For this review, take the finished solid that the model builds, in its own axes (mm). A direction names the side the tool comes from. Round coordinates to 2 decimals unless told otherwise and drop trailing zeros. Order: outer loops, then holes, each group sorted by start corner. A loop starts at its lowest first (then second) coordinate and runs counter-clockwise, first axis right, second up.
from build123d import *

# Parameters (mm, degrees)
SKETCH1_R                   = 5
SKETCH1_R_2                 = 1.15
BOSS_EXTRUDE1_DEPTH         = 1.5
FILLET1_R                   = 3
TAP_DRILL_FOR_M2_TAP1_D     = 1.6
TAP_DRILL_FOR_M2_TAP1_DEPTH = 6
TAP_DRILL_FOR_M2_TAP1_TIP   = 0.480688495
TAP_DRILL_FOR_M3_TAP1_D     = 2.5
SKETCH10_W                  = 11
SKETCH10_H                  = 2
CUT_EXTRUDE2_DEPTH          = 32.844348091
FILLET3_R                   = 0.5


with BuildPart() as part:
    # Sketch1 → Boss-Extrude1 (new, symmetric)
    with BuildSketch(Plane(origin=(0, 0, 0), x_dir=(0, 0, -1), z_dir=(1, 0, 0))):
        Polygon((-15.5, 23.75), (15.5, 23.75), (21, 23.75), (21, 20.75), (15.5, 20.75), (15.5, 8.25), (15.5, -23.75), (-15.5, -23.75), (-16.5, -23.75), (-16.5, 23.75), align=None)
        with Locations((-9, 7.422)):
            Circle(SKETCH1_R, mode=Mode.SUBTRACT)
        with Locations((-10.7, -18.75)):
            Circle(SKETCH1_R_2, mode=Mode.SUBTRACT)
        with BuildLine():
            Line((7, -4.75), (7, -14.75))
            ThreePointArc((7, -14.75), (2, -19.75), (-3, -14.75))
            Line((-3, -14.75), (-3, -4.75))
            ThreePointArc((-3, -4.75), (2, 0.25), (7, -4.75))
        make_face(mode=Mode.SUBTRACT)
    extrude(amount=BOSS_EXTRUDE1_DEPTH, both=True)

    # Fillet1
    fillet1_edges = [part.edges().sort_by_distance(p)[0] for p in [
        (0, 23.75, 16.5),
        (0, 20.75, -15.5),
    ]]
    fillet(fillet1_edges, radius=FILLET1_R)

    # Tap Drill for M2 Tap1
    with Locations(Plane(origin=(0, 23.75, 0), x_dir=(1, 0, 0), z_dir=(0, 1, 0))):
        with Locations((0, -9.5), (0, 18)):
            Hole(TAP_DRILL_FOR_M2_TAP1_D / 2, depth=TAP_DRILL_FOR_M2_TAP1_DEPTH)
            with Locations((0, 0, -(TAP_DRILL_FOR_M2_TAP1_DEPTH + TAP_DRILL_FOR_M2_TAP1_TIP / 2))):  # 118° drill point
                Cone(0, TAP_DRILL_FOR_M2_TAP1_D / 2, TAP_DRILL_FOR_M2_TAP1_TIP, mode=Mode.SUBTRACT)

    # Tap Drill for M3 Tap1 (through all)
    with Locations(Plane(origin=(1.5, 0, 0), x_dir=(0, 0, -1), z_dir=(1, 0, 0))):
        with Locations((-10.7, -11.75), (0, 18.25)):
            Hole(TAP_DRILL_FOR_M3_TAP1_D / 2)

    # Sketch10 → Cut-Extrude2 (cut, through all)
    with BuildSketch(Plane(origin=(1.5, 0, 0), x_dir=(0, 0, -1), z_dir=(1, 0, 0))):
        with Locations((0, 22.75)):
            Rectangle(SKETCH10_W, SKETCH10_H)
    extrude(amount=-CUT_EXTRUDE2_DEPTH, mode=Mode.SUBTRACT)

    # Fillet3
    fillet3_edges = [part.edges().sort_by_distance(p)[0] for p in [
        (0, 21.75, 5.5),
        (0, 23.75, 5.5),
        (0, 23.75, -5.5),
        (0, 21.75, -5.5),
    ]]
    fillet(fillet3_edges, radius=FILLET3_R)


solid = part.part
(1) Wall thickness on L1, parallel to Z at x = 1.25, y = -14.5; L2, parallel to Z at x = 0, y = 22; L3, parallel to Y at x = 0.75, z = 10.7: over which ranges is each line inside the solid? List them lowest first.
(2) Add section A-A on y = 18.25. Give the boundary of the cut face in (x, z), plus the area to 3 significant figures.
(3) Add section C-C on z = 0. Give the boundary of the cut face in (x, y), plus the area to 3 significant figures.
(4) Add section B-B on y = -6. Give the boundary of the cut face in (x, z).
(5) Add section D-D on y = -18.75. Give the boundary of the cut face in (x, z), plus the area to 3 significant figures.
(6) Tool access review of faces 4 (the face through (0, -10, -7)), 5 (the face through (-1.5, 0, 2)), 6 (the face through (0, 23, -5.5)), 7 (the face through (0, 20.75, -20)), 8 (the face through (0.104, 20.708, 8.707)): name each direction out of +Z, -Z, +X, -X, +Y, -Y from which nothing blocks a thin tool from reaching the whole face with its end or side.
(7) Draft analysis for pull direction Y (two halves, no side actions). For faces 1 (the face through (0, -23.75, 1)), 2 (the face through (0, 22, -21)), 3 (the face through (0.02, -19.75, -2.11)), state which applies: pulls with the +Y half, pulls with the -Y half, needs draft (parallel to the pull), parting line crosses it, or undercut.
(8) Clearance check with flat-ended pins moving along their axes: P1, Ø1.2, axis at x = 0.5, z = -20, coming from the -Y side; P2, Ø1.5, axis at x = -0.5, y = -9.5, coming from the -Z side. State where each tip first meets the part, or that it passes through.
Here are the results:
1. L1: z = -15.5 to -7, 3 to 16.5
1. L2: z = -21 to -18.8, -17.2 to -5.43, 5.43 to 8.7, 10.3 to 16.23
1. L3: y = -23.75 to -19.9, -17.6 to -13, -10.5 to 2.72, 12.12 to 23.75
2. outline: (-1.5, -15.54) - (1.5, -15.54) - (1.5, -1.25) - (-1.5, -1.25) - close; (-1.5, 1.25) - (1.5, 1.25) - (1.5, 16.5) - (-1.5, 16.5) - close; hole circle Ø1.6 at (0, 9.5)
2. area: 86.6 mm2
3. outline: (-1.5, -23.75) - (1.5, -23.75) - (1.5, -19.33) - (-1.5, -19.33) - close; (-1.5, -0.17) - (1.5, -0.17) - (1.5, 17) - (-1.5, 17) - close; (-1.5, 19.5) - (1.5, 19.5) - (1.5, 21.75) - (-1.5, 21.75) - close
3. area: 71.5 mm2
4. outline: (-1.5, -15.5) - (1.5, -15.5) - (1.5, -7) - (-1.5, -7) - close; (-1.5, 3) - (1.5, 3) - (1.5, 16.5) - (-1.5, 16.5) - close
5. outline: (-1.5, -15.5) - (1.5, -15.5) - (1.5, -5) - (-1.5, -5) - close; (-1.5, 1) - (1.5, 1) - (1.5, 9.55) - (-1.5, 9.55) - close; (-1.5, 11.85) - (1.5, 11.85) - (1.5, 16.5) - (-1.5, 16.5) - close
5. area: 71.1 mm2
6. face 4: +X, -X
6. face 5: +Z, -Z, -X, +Y, -Y
6. face 6: +X, -X, +Y
6. face 7: -Z, +X, -X, -Y
6. face 8: +Y
7. face 1: pulls with the -Y half
7. face 2: needs draft
7. face 3: undercut
8. P1: stops at y = 20.75
8. P2: stops at z = -15.5
